Autodesk Inventor part; units mm, degrees
ref_plane "우측면도" through (0, 0, 0) normal (1, 0, 0) x (0, 1, 0)
ref_plane "평면도" through (0, 0, 0) normal (0, 1, 0) x (-1, 0, 0)
ref_plane "정면도" through (0, 0, 0) normal (0, 0, 1) x (1, 0, 0)
sketch "스케치1" plane through (0, 0, 0) normal (0, 0, 1) x (1, 0, 0)
  circle A0 centre (0, 0) radius 98.462
  line L0 (37.6798, 90.967) -> (90.967, 37.6798)
  line L1 (90.967, 37.6798) -> (90.967, -37.6798)
  line L2 (90.967, -37.6798) -> (37.6798, -90.967)
  line L3 (37.6798, -90.967) -> (-37.6798, -90.967)
  line L4 (-37.6798, -90.967) -> (-90.967, -37.6798)
  line L5 (-90.967, -37.6798) -> (-90.967, 37.6798)
  line L6 (-90.967, 37.6798) -> (-37.6798, 90.967)
  line L7 (-37.6798, 90.967) -> (37.6798, 90.967)
  circle A1 centre (0, 0) radius 10
  dimension "d16" = 196.924
  dimension "d17" = 20
extrude "돌출1" add sketch "스케치1" against normal blind 3 contours L1 L2 L3 L4 L5 L6 L7 L0
properties part number "프레임위밑판" material "PLA 플라스틱"
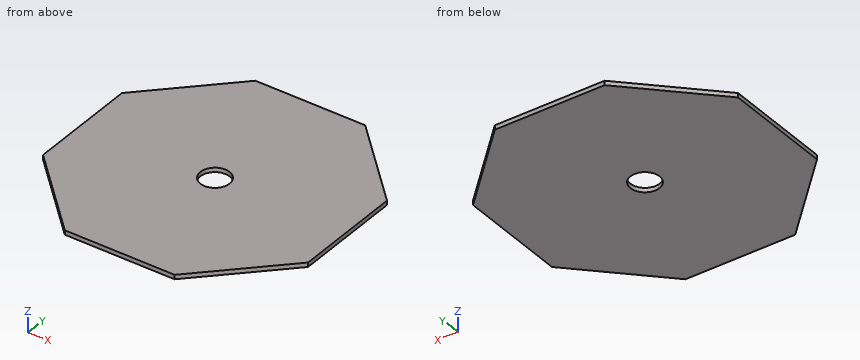
The listing builds one solid part. Answer for the finished solid, in the listing's coordinates (mm). Give positions to 0.01 mm unless a question says otherwise; leave off trailing zeros. Order: outer loops, then holes, each group sorted by start corner. A loop starts at its lowest first (then second) coordinate and runs counter-clockwise, first axis right, second up. Notation, with made-up numbers: (32, -4.75) -> (43, -4.75) arc R16 ccw to (43, 0.25) -> close; hole circle Ø11 at (40.5, 33.5). An arc over 180 degrees is marked (long way). Put each result on its own line as item: value.
Item 1: A cutting plane is placed at D-D on x = 75.5. Give the vertices of the cut face in (y, z).
Established:
outline: (-53.15, -3) -> (53.15, -3) -> (53.15, 0) -> (-53.15, 0) -> close
Item 2: A cutting plane is placed at C-C on z = -1.7. Give the vertices of the cut face in (x, y).
Established:
outline: (-90.97, -37.68) -> (-37.68, -90.97) -> (37.68, -90.97) -> (90.97, -37.68) -> (90.97, 37.68) -> (37.68, 90.97) -> (-37.68, 90.97) -> (-90.97, 37.68) -> close; hole circle Ø20 at (0, 0)
Item 3: Given P1, Ø6, axis at x = 67.5, y = -41.5, coming from the +Z side, flat-ended and moving along its own axis, determine where the tip first touches the part or whether it passes through.
Established:
P1: stops at z = 0
Item 4: Straight lines are drawn through the part: line 1 (Y direction, x = 0, z = -0.85); line 2 (Y direction, x = -7.5, z = -0.6); line 3 (X direction, y = 6, z = -2.6). For each, find the intervals that lie inside material, in ascending order.
Established:
line 1: y = -90.97 to -10, 10 to 90.97
line 2: y = -90.97 to -6.61, 6.61 to 90.97
line 3: x = -90.97 to -8, 8 to 90.97
Item 5: A cutting plane is placed at A-A on x = 0. Give the vertices of the cut face in (y, z), plus the area to 3 significant figures.
Established:
outline: (-90.97, -3) -> (-10, -3) -> (-10, 0) -> (-90.97, 0) -> close; (10, -3) -> (90.97, -3) -> (90.97, 0) -> (10, 0) -> close
area: 486 mm^2
